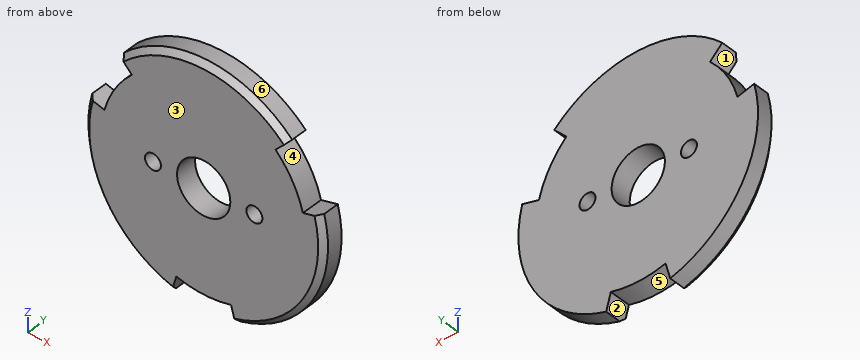
from build123d import *

# Parameters (mm, degrees)
SKETCH1_R           = 22.5
SKETCH1_R_2         = 5
SKETCH1_R_3         = 1.5
BOSS_EXTRUDE1_DEPTH = 4
CHAMFER1_SIZE       = 1
CUT_EXTRUDE1_DEPTH  = 5


with BuildPart() as part:
    # Sketch1 → Boss-Extrude1 (new body)
    with BuildSketch(Plane(origin=(0, 0, 0), x_dir=(1, 0, 0), z_dir=(0, 1, 0))):
        Circle(SKETCH1_R)
        Circle(SKETCH1_R_2, mode=Mode.SUBTRACT)
        with Locations((-9.525, 0)):
            Circle(SKETCH1_R_3, mode=Mode.SUBTRACT)
        with Locations((9.525, 0)):
            Circle(SKETCH1_R_3, mode=Mode.SUBTRACT)
    extrude(amount=BOSS_EXTRUDE1_DEPTH)

    # Chamfer1
    chamfer1_edges = [part.edges().sort_by_distance(p)[0] for p in [
        (-22.5, 0, 0),
    ]]
    chamfer(chamfer1_edges, length=CHAMFER1_SIZE)

    # Sketch2 → Cut-Extrude1 (cut, through all)
    with BuildSketch(Plane(origin=(0, 4, 0), x_dir=(1, 0, 0), z_dir=(0, 1, 0))):
        with BuildLine():
            Line((6.012863462, 21.681685197), (5.14433874, 18.549886224))
            ThreePointArc((5.14433874, 18.549886224), (0, 19.25), (-5.14433874, 18.549886224))
            Line((-5.14433874, 18.549886224), (-6.012863462, 21.681685197))
            ThreePointArc((-6.012863462, 21.681685197), (0, 22.5), (6.012863462, 21.681685197))
        make_face()
        with BuildLine():
            Line((21.783321909, -5.633550091), (18.636842077, -4.819815078))
            ThreePointArc((18.636842077, -4.819815078), (16.670989023, -9.625), (13.492503338, -13.730071146))
            Line((13.492503338, -13.730071146), (15.770458447, -16.048135106))
            ThreePointArc((15.770458447, -16.048135106), (19.485571585, -11.25), (21.783321909, -5.633550091))
        make_face()
        with BuildLine():
            Line((-15.770458447, -16.048135106), (-13.492503338, -13.730071146))
            ThreePointArc((-13.492503338, -13.730071146), (-16.670989023, -9.625), (-18.636842077, -4.819815078))
            Line((-18.636842077, -4.819815078), (-21.783321909, -5.633550091))
            ThreePointArc((-21.783321909, -5.633550091), (-19.485571585, -11.25), (-15.770458447, -16.048135106))
        make_face()
    extrude(amount=-CUT_EXTRUDE1_DEPTH, mode=Mode.SUBTRACT)


solid = part.part
Can you work these out from the model? Positions are in its coordinate system, mm. Face numbers are marked on the shaded views. A direction names the side the tool comes from. Round coordinates to 2 decimals unless told otherwise and drop trailing zeros. Write each loop counter-clockwise with the first axis right and the second up, starting at its lowest first coordinate (ties: lowest second). Pieces come first, ordered by that corner, then holes. Notation, with made-up numbers: M 84.25,52 L 96.25,52 A31 ccw 96.25,77 Z; hole C 89.5,77.25 d4. An arc over 180 degrees is marked long. Use CSV: the item, a comma, the result in double quotes.
(1) I need wall thicknesses on line 1 along X through (y, z) = (1.7, 0) (3 decimals); line 2 along Z through (x, y) = (0, 2.4); line 3 along X through (y, z) = (3.3, 2). Which ranges of each line are inside material? Lowest first, please.
Check values:
line 1,"-22.5 to -11.025, -8.025 to -5, 5 to 8.025, 11.025 to 22.5"
line 2,"-19.25 to -5, 5 to 22.5"
line 3,"-22.41 to -4.58, 4.58 to 22.41"
(2) Imagine slicing it at B-B (z = 0). Write out the boundary of the cut face in (x, y) (3 decimals).
Check values:
outline,"M -22.5,1 L -21.5,0 L -11.025,0 L -11.025,4 L -22.5,4 Z; M -8.025,0 L -5,0 L -5,4 L -8.025,4 Z; M 5,0 L 8.025,0 L 8.025,4 L 5,4 Z; M 11.025,0 L 21.5,0 L 22.5,1 L 22.5,4 L 11.025,4 Z"
(3) Imagine slicing it at C-C (y = 1.85). Count the separate pieces of the cut face and the enclosed holes in it, plus the area to 3 significant figures.
Check values:
separate pieces,"1"
enclosed holes,"3"
area,"1,390 mm^2"
(4) Imagine slicing it at A-A (x = 0). Write out the boundary of the cut face in (y, z), plus the area to 4 significant figures.
Check values:
outline,"M 0,-19.25 L 4,-19.25 L 4,-5 L 0,-5 Z; M 0,5 L 4,5 L 4,22.5 L 1,22.5 L 0,21.5 Z"
area,"126.5 mm^2"
(5) On a 3-axis mill with a long thin cutter (end or side, diameter ignored), from which of +Z, -Z, +X, -X, +Y, -Y can I reach the whole of each face in a straight line? I mean the marked faces 1, 2 and 3. Say none if no direction works.
Check values:
face 1,"-X, +Y, -Y"
face 2,"-Z, +Y, -Y"
face 3,"+Z, -Z, +X, -X, -Y"
(6) I'm going to push flat-ended pins straight in: pin 1 (12 mm diameter, centred on x = -4.5, z = 1.5, fed in from +Y); pin 2 (1 mm diameter, centred on x = 11.5, y = 3.5, fed in from +Z). Where does each tip first touch, or does it pass through?
Check values:
pin 1,"y = 4"
pin 2,"z = 19.63"
(7) Imagine slicing it at D-D (z = 14.5). Write out the boundary of the cut face in (x, y), plus the area to 3 significant figures.
Check values:
outline,"M -14.25,0 L 14.25,0 L 14.25,4 L -14.25,4 Z"
area,"114 mm^2"
(8) We'd pull the mould along Z, two halves only. Please class the marked faces 4, 5 and 6: +Z half, -Z half, draft (parallel to the pull), parting line (faces both ways), or undercut.
Check values:
face 4,"undercut"
face 5,"-Z half"
face 6,"+Z half"
